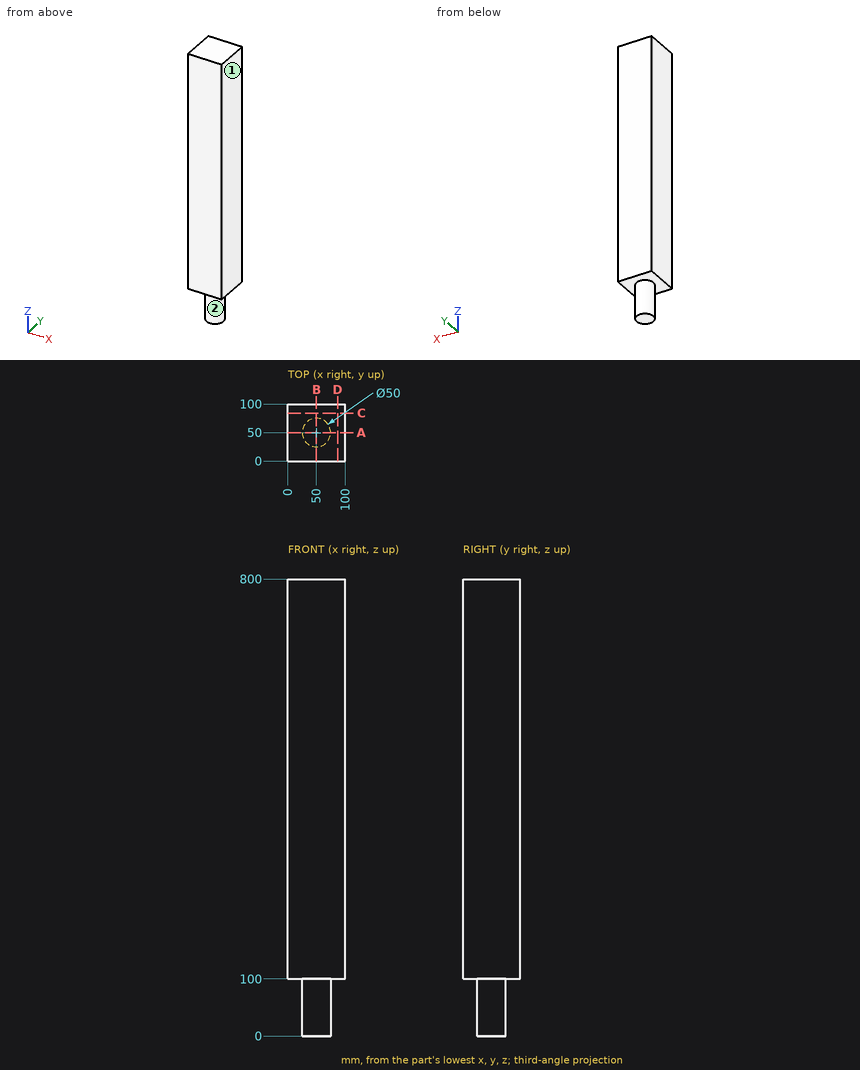
Check sheet for the drawn part. Datum: minimum x, y, z corner. Units: mm. A direction names the side the tool comes from. Round coordinates to 2 decimals unless told otherwise and drop trailing zeros. Write each loop counter-clockwise with the first axis right and the second up, starting at its lowest first coordinate (ties: lowest second). Pieces come first, ordered by that corner, then holes. Notation, with made-up numbers: (-12, 37) -> (32, 37) arc R26 cw to (32, 70) -> close; hole circle Ø10 at (86, 78.25). An arc over 180 degrees is marked (long way). One line per item, written item: value. Start each with the question number.
(1) Scan line: line 1 (Z direction, x = 93, y = 53). Record every from-to range of solid material in increasing order. Write a range as [from, to].
(2) Cross-section at C-C, the plane y = 84. Record the cut outline in (x, z).
(3) Go/stop test with a flat-tipped pin: pin 1 Ø2 at (x, y) = (22.5, 85) entering from -Z. Record where the tip stops, or that it passes through.
(4) Cross-section at A-A, the plane y = 50. Record the cut outline in (x, z).
(5) Access from +Z, -Z, +X, -X, +Y, -Y to the whole of each face (thin tool, end or side, straight path). Record for the marked faces 1 and 2.
Answer:
1. line 1: [100, 800]
2. outline: (0, 100) -> (100, 100) -> (100, 800) -> (0, 800) -> close
3. pin 1: z = 100
4. outline: (0, 100) -> (25, 100) -> (25, 0) -> (75, 0) -> (75, 100) -> (100, 100) -> (100, 800) -> (0, 800) -> close
5. face 1: +Z, -Z, +X, +Y, -Y
5. face 2: -Z
